Check sheet for the modelled part. Datum: model origin and axes. Units: mm. A direction names the side the tool comes from. Round coordinates to 2 decimals unless told otherwise and drop trailing zeros. Loops run counter-clockwise (first coordinate to the right, second up) from the corner with the lowest first, then second, coordinate; pieces in that order, holes last. Notation, with made-up numbers: (11, 73) -> (29, 73) arc R11 cw to (29, 77) -> close; hole circle Ø10 at (-1, -26.5). An arc over 180 degrees is marked (long way). Return JSON: item names as keys, results as strings.
from build123d import *

# Parameters (mm, degrees)
BOSS_EXTRUDE1_DEPTH                           = 3
CSK_FOR_M3_COUNTERSUNK_FLAT_HEAD_SCR_2_COUNT  = 2
CSK_FOR_M3_COUNTERSUNK_FLAT_HEAD_SCR_2_PITCH  = 90
CSK_FOR_M3_COUNTERSUNK_FLAT_HEAD_SCR_3_COUNT  = 2
CSK_FOR_M3_COUNTERSUNK_FLAT_HEAD_SCR_3_PITCH  = 138.676782484
CSK_FOR_M3_COUNTERSUNK_FLAT_HEAD_SCR_4_COUNT  = 2
CSK_FOR_M3_COUNTERSUNK_FLAT_HEAD_SCR_4_PITCH  = 72.672209269
CSK_FOR_M3_COUNTERSUNK_FLAT_HEAD_SCR_5_COUNT  = 2
CSK_FOR_M3_COUNTERSUNK_FLAT_HEAD_SCR_5_PITCH  = 133.375410027
CSK_FOR_M3_COUNTERSUNK_FLAT_HEAD_SCR_6_COUNT  = 2
CSK_FOR_M3_COUNTERSUNK_FLAT_HEAD_SCR_6_PITCH  = 155.206314305
CSK_FOR_M3_COUNTERSUNK_FLAT_HEAD_SCR_7_COUNT  = 2
CSK_FOR_M3_COUNTERSUNK_FLAT_HEAD_SCR_7_PITCH  = 102
CSK_FOR_M3_COUNTERSUNK_FLAT_HEAD_SCR_8_COUNT  = 2
CSK_FOR_M3_COUNTERSUNK_FLAT_HEAD_SCR_8_PITCH  = 126.035709226
CSK_FOR_M3_COUNTERSUNK_FLAT_HEAD_SCR_9_COUNT  = 2
CSK_FOR_M3_COUNTERSUNK_FLAT_HEAD_SCR_9_PITCH  = 160.240444333
CSK_FOR_M3_COUNTERSUNK_FLAT_HEAD_SCR_10_COUNT = 2
CSK_FOR_M3_COUNTERSUNK_FLAT_HEAD_SCR_10_PITCH = 77.620873481
CSK_FOR_M3_COUNTERSUNK_FLAT_HEAD_SCR_11_COUNT = 2
CSK_FOR_M3_COUNTERSUNK_FLAT_HEAD_SCR_11_PITCH = 149.48244044
CSK_FOR_M3_COUNTERSUNK_FLAT_HEAD_SCR_12_COUNT = 2
CSK_FOR_M3_COUNTERSUNK_FLAT_HEAD_SCR_12_PITCH = 73.246160309
CSK_FOR_M3_COUNTERSUNK_FLAT_HEAD_SCR_13_COUNT = 2
CSK_FOR_M3_COUNTERSUNK_FLAT_HEAD_SCR_13_PITCH = 130.357201566
CSK_FOR_M3_COUNTERSUNK_FLAT_HEAD_SCR_14_COUNT = 2
CSK_FOR_M3_COUNTERSUNK_FLAT_HEAD_SCR_14_PITCH = 142.523682243
CSK_FOR_M3_COUNTERSUNK_FLAT_HEAD_SCR_15_COUNT = 2
CSK_FOR_M3_COUNTERSUNK_FLAT_HEAD_SCR_15_PITCH = 75
SKETCH14_W                                    = 60
SKETCH14_H                                    = 20
CUT_EXTRUDE1_DEPTH                            = 123.366253518
FILLET1_R                                     = 3
BOSS_EXTRUDE3_REACH                           = 115.874
SKETCH21_W                                    = 12
SKETCH21_H                                    = 12
SKETCH21_R                                    = 4
SKETCH21_2_W                                  = 12
SKETCH21_2_H                                  = 12
CUT_EXTRUDE3_DEPTH                            = 29
FILLET2_R                                     = 4
FILLET3_R                                     = 1


with BuildPart() as part:
    # Sketch1 → Boss-Extrude1 (new body)
    with BuildSketch(Plane(origin=(0, 0, 0), x_dir=(1, 0, 0), z_dir=(0, 1, 0))):
        with BuildLine():
            Line((-52.657863609, 68.625063935), (52.657863609, 68.625063935))
            ThreePointArc((52.657863609, 68.625063935), (0, -86.5), (-52.657863609, 68.625063935))
        make_face()
    extrude(amount=BOSS_EXTRUDE1_DEPTH)

    # Sketch9 → CSK for M3 Countersunk Flat Head Screw3 (revolve, cut)
    with BuildSketch(Plane(origin=(-45, 3, -63), x_dir=(0, 0, 1), z_dir=(1, 0, 0))):
        Polygon((0, 0), (0, 3), (1.8, 3), (1.8, 1.35), (3.15, 0), align=None)
    csk_for_m3_countersunk_flat_head_screw3 = revolve(axis=Axis((-45, 9.35, -63), (0, -1, 0)), mode=Mode.SUBTRACT)

    # CSK for M3 Countersunk Flat Head Scr 2: CSK for M3 Countersunk Flat Head Screw3 ×2
    with Locations(*[(i * CSK_FOR_M3_COUNTERSUNK_FLAT_HEAD_SCR_2_PITCH, 0, 0) for i in range(1, CSK_FOR_M3_COUNTERSUNK_FLAT_HEAD_SCR_2_COUNT)]):
        add(csk_for_m3_countersunk_flat_head_screw3, mode=Mode.SUBTRACT)

    # CSK for M3 Countersunk Flat Head Scr 3: CSK for M3 Countersunk Flat Head Screw3 ×2
    with Locations(*[Vector(0.8833490206949295, 0, 0.46871580689935033) * (i * CSK_FOR_M3_COUNTERSUNK_FLAT_HEAD_SCR_3_PITCH) for i in range(1, CSK_FOR_M3_COUNTERSUNK_FLAT_HEAD_SCR_3_COUNT)]):
        add(csk_for_m3_countersunk_flat_head_screw3, mode=Mode.SUBTRACT)

    # CSK for M3 Countersunk Flat Head Scr 4: CSK for M3 Countersunk Flat Head Screw3 ×2
    with Locations(*[Vector(-0.4472135954999581, 0, 0.894427190999916) * (i * CSK_FOR_M3_COUNTERSUNK_FLAT_HEAD_SCR_4_PITCH) for i in range(1, CSK_FOR_M3_COUNTERSUNK_FLAT_HEAD_SCR_4_COUNT)]):
        add(csk_for_m3_countersunk_flat_head_screw3, mode=Mode.SUBTRACT)

    # CSK for M3 Countersunk Flat Head Scr 5: CSK for M3 Countersunk Flat Head Screw3 ×2
    with Locations(*[Vector(0.07497633932626105, 0, 0.9971853130392733) * (i * CSK_FOR_M3_COUNTERSUNK_FLAT_HEAD_SCR_5_PITCH) for i in range(1, CSK_FOR_M3_COUNTERSUNK_FLAT_HEAD_SCR_5_COUNT)]):
        add(csk_for_m3_countersunk_flat_head_screw3, mode=Mode.SUBTRACT)

    # CSK for M3 Countersunk Flat Head Scr 6: CSK for M3 Countersunk Flat Head Screw3 ×2
    with Locations(*[Vector(0.5154429467542566, 0, 0.8569238989789517) * (i * CSK_FOR_M3_COUNTERSUNK_FLAT_HEAD_SCR_6_PITCH) for i in range(1, CSK_FOR_M3_COUNTERSUNK_FLAT_HEAD_SCR_6_COUNT)]):
        add(csk_for_m3_countersunk_flat_head_screw3, mode=Mode.SUBTRACT)

    # Sketch13 → CSK for M3 Countersunk Flat Head Screw4 (revolve, cut)
    with BuildSketch(Plane(origin=(-51, 0, -61), x_dir=(0, 0, -1), z_dir=(1, 0, 0))):
        Polygon((0, 0), (0, 3), (1.8, 3), (1.8, 1.35), (3.15, 0), align=None)
    csk_for_m3_countersunk_flat_head_screw4 = revolve(axis=Axis((-51, -6.35, -61), (0, 1, 0)), mode=Mode.SUBTRACT)

    # CSK for M3 Countersunk Flat Head Scr 7: CSK for M3 Countersunk Flat Head Screw4 ×2
    with Locations(*[(i * CSK_FOR_M3_COUNTERSUNK_FLAT_HEAD_SCR_7_PITCH, 0, 0) for i in range(1, CSK_FOR_M3_COUNTERSUNK_FLAT_HEAD_SCR_7_COUNT)]):
        add(csk_for_m3_countersunk_flat_head_screw4, mode=Mode.SUBTRACT)

    # CSK for M3 Countersunk Flat Head Scr 8: CSK for M3 Countersunk Flat Head Screw4 ×2
    with Locations(*[Vector(0.023802777946288843, 0, 0.9997166737441362) * (i * CSK_FOR_M3_COUNTERSUNK_FLAT_HEAD_SCR_8_PITCH) for i in range(1, CSK_FOR_M3_COUNTERSUNK_FLAT_HEAD_SCR_8_COUNT)]):
        add(csk_for_m3_countersunk_flat_head_screw4, mode=Mode.SUBTRACT)

    # CSK for M3 Countersunk Flat Head Scr 9: CSK for M3 Countersunk Flat Head Screw4 ×2
    with Locations(*[Vector(0.6178215519319036, 0, 0.7863183388224227) * (i * CSK_FOR_M3_COUNTERSUNK_FLAT_HEAD_SCR_9_PITCH) for i in range(1, CSK_FOR_M3_COUNTERSUNK_FLAT_HEAD_SCR_9_COUNT)]):
        add(csk_for_m3_countersunk_flat_head_screw4, mode=Mode.SUBTRACT)

    # CSK for M3 Countersunk Flat Head Scr 10: CSK for M3 Countersunk Flat Head Screw4 ×2
    with Locations(*[Vector(-0.373610843312482, 0, 0.9275855420171965) * (i * CSK_FOR_M3_COUNTERSUNK_FLAT_HEAD_SCR_10_PITCH) for i in range(1, CSK_FOR_M3_COUNTERSUNK_FLAT_HEAD_SCR_10_COUNT)]):
        add(csk_for_m3_countersunk_flat_head_screw4, mode=Mode.SUBTRACT)

    # CSK for M3 Countersunk Flat Head Scr 11: CSK for M3 Countersunk Flat Head Screw4 ×2
    with Locations(*[Vector(0.8763571133445796, 0, 0.4816619248916773) * (i * CSK_FOR_M3_COUNTERSUNK_FLAT_HEAD_SCR_11_PITCH) for i in range(1, CSK_FOR_M3_COUNTERSUNK_FLAT_HEAD_SCR_11_COUNT)]):
        add(csk_for_m3_countersunk_flat_head_screw4, mode=Mode.SUBTRACT)

    # CSK for M3 Countersunk Flat Head Scr 12: CSK for M3 Countersunk Flat Head Screw4 ×2
    with Locations(*[Vector(-0.08191555672945391, 0, 0.996639273541688) * (i * CSK_FOR_M3_COUNTERSUNK_FLAT_HEAD_SCR_12_PITCH) for i in range(1, CSK_FOR_M3_COUNTERSUNK_FLAT_HEAD_SCR_12_COUNT)]):
        add(csk_for_m3_countersunk_flat_head_screw4, mode=Mode.SUBTRACT)

    # CSK for M3 Countersunk Flat Head Scr 13: CSK for M3 Countersunk Flat Head Screw4 ×2
    with Locations(*[Vector(0.8284927775601016, 0, 0.559999747795254) * (i * CSK_FOR_M3_COUNTERSUNK_FLAT_HEAD_SCR_13_PITCH) for i in range(1, CSK_FOR_M3_COUNTERSUNK_FLAT_HEAD_SCR_13_COUNT)]):
        add(csk_for_m3_countersunk_flat_head_screw4, mode=Mode.SUBTRACT)

    # CSK for M3 Countersunk Flat Head Scr 14: CSK for M3 Countersunk Flat Head Screw4 ×2
    with Locations(*[Vector(0.8630144693469346, 0, 0.5051792015689374) * (i * CSK_FOR_M3_COUNTERSUNK_FLAT_HEAD_SCR_14_PITCH) for i in range(1, CSK_FOR_M3_COUNTERSUNK_FLAT_HEAD_SCR_14_COUNT)]):
        add(csk_for_m3_countersunk_flat_head_screw4, mode=Mode.SUBTRACT)

    # CSK for M3 Countersunk Flat Head Scr 15: CSK for M3 Countersunk Flat Head Screw4 ×2
    with Locations(*[Vector(-0.2800000000000003, 0, 0.96) * (i * CSK_FOR_M3_COUNTERSUNK_FLAT_HEAD_SCR_15_PITCH) for i in range(1, CSK_FOR_M3_COUNTERSUNK_FLAT_HEAD_SCR_15_COUNT)]):
        add(csk_for_m3_countersunk_flat_head_screw4, mode=Mode.SUBTRACT)

    # Sketch14 → Cut-Extrude1 (cut, through all)
    with BuildSketch(Plane(origin=(0, 3, 0), x_dir=(1, 0, 0), z_dir=(0, 1, 0))):
        with BuildLine():
            Line((65.926094985, 56), (45, 56))
            Line((45, 56), (45, 5))
            Line((45, 5), (45, -6.5))
            Line((45, -6.5), (69, -6.5))
            Line((69, -6.5), (69, 5))
            Line((69, 5), (86.355370418, 5))
            ThreePointArc((86.355370418, 5), (80.297329821, 32.165024851), (65.926094985, 56))
        make_face()
        with BuildLine():
            Line((64.5, -17), (45, -17))
            Line((45, -17), (45, -59))
            Line((45, -59), (63.255434549, -59))
            ThreePointArc((63.255434549, -59), (73.067302991, -46.297075864), (80.363237864, -32))
            Line((80.363237864, -32), (64.5, -32))
            Line((64.5, -32), (64.5, -17))
        make_face()
        with BuildLine():
            Line((-45, -59), (-63.255434549, -59))
            ThreePointArc((-63.255434549, -59), (-73.067302991, -46.297075864), (-80.363237864, -32))
            ThreePointArc((-80.363237864, -32), (-82.927979827, -24.600816282), (-84.813029659, -17))
            Line((-84.813029659, -17), (-64.5, -17))
            Line((-64.5, -17), (-45, -17))
            Line((-45, -17), (-45, -59))
        make_face()
        with BuildLine():
            Line((-69, 5), (-86.355370418, 5))
            ThreePointArc((-86.355370418, 5), (-80.297329821, 32.165024851), (-65.926094985, 56))
            Line((-65.926094985, 56), (-45, 56))
            Line((-45, 56), (-45, 5))
            Line((-45, 5), (-45, -6.5))
            Line((-45, -6.5), (-69, -6.5))
            Line((-69, -6.5), (-69, 5))
        make_face()
        with Locations((0, 50.625063935)):
            Rectangle(SKETCH14_W, SKETCH14_H)
        with BuildLine():
            Line((44.791182168, -74), (27.5, -74))
            Line((27.5, -74), (27.5, -68))
            Line((27.5, -68), (-27.5, -68))
            Line((-27.5, -68), (-27.5, -74))
            Line((-27.5, -74), (-44.791182168, -74))
            ThreePointArc((-44.791182168, -74), (0, -86.5), (44.791182168, -74))
        make_face()
    extrude(amount=-CUT_EXTRUDE1_DEPTH, mode=Mode.SUBTRACT)

    # Fillet1
    fillet1_edges = [part.edges().sort_by_distance(p)[0] for p in [
        (65.926094985, 1.5, -56),
        (45, 1.5, -56),
        (86.355370418, 1.5, -5),
        (45, 1.5, 17),
        (45, 1.5, 59),
        (63.255434549, 1.5, 59),
        (-63.255434549, 1.5, 59),
        (-45, 1.5, 59),
        (-84.813029659, 1.5, 17),
        (-45, 1.5, 17),
        (-86.355370418, 1.5, -5),
        (-65.926094985, 1.5, -56),
        (-45, 1.5, -56),
        (-30, 1.5, -40.625063935),
        (-30, 1.5, -60.625063935),
        (30, 1.5, -40.625063935),
        (30, 1.5, -60.625063935),
        (80.363237864, 1.5, 32),
        (64.5, 1.5, 32),
        (64.5, 1.5, 17),
        (-52.657863609, 1.5, -68.625063935),
        (52.657863609, 1.5, -68.625063935),
        (44.791182168, 1.5, 74),
        (-27.5, 1.5, 74),
        (-27.5, 1.5, 68),
        (27.5, 1.5, 68),
        (27.5, 1.5, 74),
        (-44.791182168, 1.5, 74),
        (-69, 1.5, 6.5),
        (-69, 1.5, -5),
        (-45, 1.5, 6.5),
        (69, 1.5, -5),
        (69, 1.5, 6.5),
        (45, 1.5, 6.5),
    ]]
    fillet(fillet1_edges, radius=FILLET1_R - 0.0001)  # a hair under: the kernel refuses the full size

    # Boss-Extrude3: up to this face of the body (flat: up to its plane)
    boss_extrude3_end = Plane(part.part.faces().sort_by_distance((72.901134209, 1.5, 32))[0])
    # Sketch21 → Boss-Extrude3 (add, up to the picked face)
    with BuildSketch(Plane.XY, mode=Mode.PRIVATE) as boss_extrude3_sk1:
        with Locations((73.5, -6)):
            Rectangle(SKETCH21_W, SKETCH21_H)
        with Locations(Location((73.5, -6, 0), (0, 0, 180))):
            Circle(SKETCH21_R, mode=Mode.SUBTRACT)
    boss_extrude3_tool1 = split(extrude(boss_extrude3_sk1.sketch, amount=BOSS_EXTRUDE3_REACH, mode=Mode.PRIVATE), bisect_by=boss_extrude3_end, keep=Keep.BOTH, mode=Mode.PRIVATE)
    add(boss_extrude3_tool1.solids().sort_by(Axis((73.5, -0.169706, 0), (0, 0, 1)))[0])

    # Sketch21<2> → Cut-Extrude3 (cut)
    with BuildSketch(Plane.XY):
        with Locations((73.5, -6)):
            Rectangle(SKETCH21_2_W, SKETCH21_2_H)
    extrude(amount=CUT_EXTRUDE3_DEPTH, mode=Mode.SUBTRACT)

    # Fillet2
    fillet2_edges = [part.edges().sort_by_distance(p)[0] for p in [
        (79.5, -12, 30.5),
        (67.5, -12, 30.5),
    ]]
    fillet(fillet2_edges, radius=FILLET2_R)

    # Fillet3
    fillet3_edges = [part.edges().sort_by_distance(p)[0] for p in [
        (79.5, 0, 30.375284399),
        (67.5, 0, 30.5),
        (77.5, -6, 29),
    ]]
    fillet(fillet3_edges, radius=FILLET3_R)


solid = part.part
Q1. Draft check along Z on faces 3 (the cylindrical face through (52.03, 1.48, 69.1)), 4 (the cylindrical face through (58.597, 2.163, 11.169)), 5 (the cylindrical face through (-57.5, 1.48, -64.62)), 6 (the cylindrical face through (77.496, -6.176, 30.986)). Enter one of: released by +Z, released by -Z, zero draft, split by the parting line, or undercut.
Results list:
{"face 3": "released by +Z", "face 4": "undercut", "face 5": "released by -Z", "face 6": "zero draft"}
Q2. Material ranges on line 1 (X direction, y = 0.95, z = 70); line 2 (X direction, y = 2.5, z = -61); line 3 (Z direction, x = -51, y = 2.05), recorded low to high.
Results list:
{"line 1": "-50.82 to -36.8, -33.2 to -27.33, 27.33 to 33.2, 36.8 to 50.82", "line 2": "-61.32 to -52.8, -49.2 to -46.74, -43.26 to 43.26, 46.74 to 49.2, 52.8 to 61.32", "line 3": "-68.63 to -62.8, -59.2 to -56, 6.5 to 17, 59 to 69.87"}
Q3. Section check A-A (x = 5). Record the boundary of the cut face in (y, z).
Results list:
{"outline": "(0, -68.63) -> (3, -68.63) -> (3, -60.63) -> (0, -60.63) -> close; (0, -40.63) -> (3, -40.63) -> (3, 68) -> (0, 68) -> close"}
Q4. Tool access check on faces 1 (the cylindrical face through (81.757, 2.163, 11.39)), 2 (the flat face through (74, -1, 32)). Record the directions out of +Z, -Z, +X, -X, +Y, -Y that give a thin tool (end or side, any length) a straight path to the whole face; none if there is none.
Results list:
{"face 1": "+Y, -Y", "face 2": "+Z, +X, +Y, -Y"}
Q5. Section check B-B (z = 25.5). Record the boundary of the cut face in (x, y), then the cut area to 3 significant figures.
Results list:
{"outline": "(-45, 0) -> (45, 0) -> (45, 3) -> (-45, 3) -> close; (64.5, 0) -> (82.66, 0) -> (82.66, 3) -> (64.5, 3) -> close", "area": "324 mm^2"}
Q6. Go/stop test with flat-tipped pins: pin 1 (0.9 mm diameter, centred on y = -2.5, z = 30.5, fed in from +X); pin 2 (2.5 mm diameter, centred on x = 55.5, y = 2, fed in from +Z); pin 3 (4 mm diameter, centred on x = 72, z = 11, fed in from -Y). Record where each tip stops, or that it passes through.
Results list:
{"pin 1": "x = 79.5", "pin 2": "z = 67.37", "pin 3": "y = 1.15"}
